Build history of the part. All positions in model axes, mm. Round coordinates to 2 decimals unless told otherwise and drop trailing zeros. Loops run counter-clockwise (first coordinate to the right, second up) from the corner with the lowest first, then second, coordinate; pieces in that order, holes last.
from build123d import *

# Parameters (mm, degrees)
SM_BASE_FLANGE_1_DEPTH      = 1.5
HOLE_WIZARD_M3_1_AT_2_COUNT = 2
HOLE_WIZARD_M3_1_AT_2_PITCH = 60
HOLE_WIZARD_M3_1_AT_3_COUNT = 2
HOLE_WIZARD_M3_1_AT_3_PITCH = 84.852813742
HOLE_WIZARD_M3_1_AT_4_COUNT = 2
HOLE_WIZARD_M3_1_AT_4_PITCH = 60
HOLE_WIZARD_1_D             = 28
HOLE_WIZARD_1_DEPTH         = 100
HOLE_WIZARD_M4_1_D          = 3.3
PATTERN_CIRCULAR_1_COUNT    = 4


# Sheet-metal steps are written as plain solids
with BuildPart() as part:
    # Sketch 1 → 基体-法兰1 (new body)
    with BuildSketch(Plane(origin=(0, 0, 0), x_dir=(0, 0, -1), z_dir=(1, 0, 0))):
        with BuildLine():
            Line((-30, -50), (30, -50))
            ThreePointArc((30, -50), (44.142135624, -44.142135624), (50, -30))
            Line((50, -30), (50, 30))
            ThreePointArc((50, 30), (44.142135624, 44.142135624), (30, 50))
            Line((30, 50), (-30, 50))
            ThreePointArc((-30, 50), (-44.142135624, 44.142135624), (-50, 30))
            Line((-50, 30), (-50, -30))
            ThreePointArc((-50, -30), (-44.142135624, -44.142135624), (-30, -50))
        make_face()
    extrude(amount=-SM_BASE_FLANGE_1_DEPTH)

    # 草图4 → M3 六角凹锥坑头螺钉的锥形沉头孔1 (revolve, cut)
    with BuildSketch(Plane(origin=(-1.5, 30, -30), x_dir=(0, 0, 1), z_dir=(0, 1, 0))):
        Polygon((0, 0), (0, 1.5), (1.7, 1.5), (1.7, 1.77), (3.47, 0), align=None)
    hole_wizard_m3_1 = revolve(axis=Axis((-7.85, 30, -30), (1, 0, 0)), mode=Mode.SUBTRACT)

    # M3 六角凹锥坑头螺钉的锥形沉头孔1 at 2: M3 六角凹锥坑头螺钉的锥形沉头孔1 ×2
    with Locations(*[(0, 0, i * HOLE_WIZARD_M3_1_AT_2_PITCH) for i in range(1, HOLE_WIZARD_M3_1_AT_2_COUNT)]):
        add(hole_wizard_m3_1, mode=Mode.SUBTRACT)

    # M3 六角凹锥坑头螺钉的锥形沉头孔1 at 3: M3 六角凹锥坑头螺钉的锥形沉头孔1 ×2
    with Locations(*[Vector(0, -0.7071067811865476, 0.7071067811865476) * (i * HOLE_WIZARD_M3_1_AT_3_PITCH) for i in range(1, HOLE_WIZARD_M3_1_AT_3_COUNT)]):
        add(hole_wizard_m3_1, mode=Mode.SUBTRACT)

    # M3 六角凹锥坑头螺钉的锥形沉头孔1 at 4: M3 六角凹锥坑头螺钉的锥形沉头孔1 ×2
    with Locations(*[(0, -i * HOLE_WIZARD_M3_1_AT_4_PITCH, 0) for i in range(1, HOLE_WIZARD_M3_1_AT_4_COUNT)]):
        add(hole_wizard_m3_1, mode=Mode.SUBTRACT)

    # 孔1
    with Locations(Plane.ZY.offset(1.5)):
        with Locations((0, 0)):
            Hole(HOLE_WIZARD_1_D / 2, depth=HOLE_WIZARD_1_DEPTH)

    # M4 螺纹孔1 (through all)
    with Locations(Plane.ZY.offset(1.5)):
        with Locations((0, 27.5)):
            hole_wizard_m4_1 = Hole(HOLE_WIZARD_M4_1_D / 2)

    # 阵列(圆周)1: M4 螺纹孔1 ×4 about axis
    pattern_circular_1_axis = Axis((0, 0, 0), (1, 0, 0))
    for i in range(1, PATTERN_CIRCULAR_1_COUNT):
        add(hole_wizard_m4_1.rotate(pattern_circular_1_axis, i * 360 / PATTERN_CIRCULAR_1_COUNT), mode=Mode.SUBTRACT)


solid = part.part
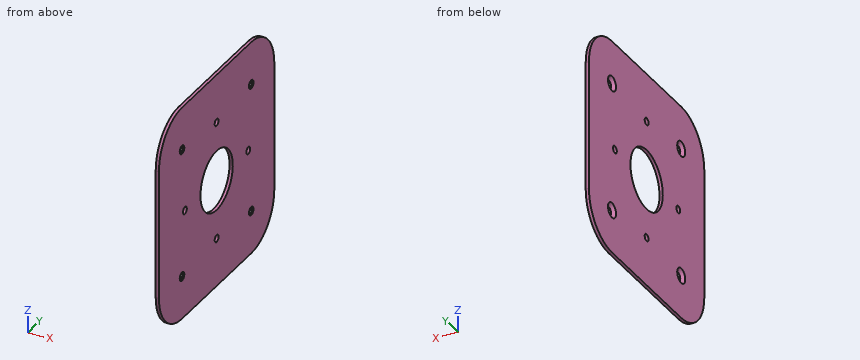
(1) Slice it at A-A on y = 0. List the corners of the cut face in (x, z).
Responses:
outline: (-1.5, -50) - (0, -50) - (0, -29.15) - (-1.5, -29.15) - close; (-1.5, -25.85) - (0, -25.85) - (0, -14) - (-1.5, -14) - close; (-1.5, 14) - (0, 14) - (0, 25.85) - (-1.5, 25.85) - close; (-1.5, 29.15) - (0, 29.15) - (0, 50) - (-1.5, 50) - close
(2) Slice it at C-C on x = -1.25. Count the separate pieces of the cut face and the enclosed holes in it, plus the area to 3 significant figures.
Responses:
separate pieces: 1
enclosed holes: 9
area: 8,880 mm2
(3) Probe line 1 (Y direction, x = -0.5, z = 0); line 2 (Y direction, x = -0.35, z = -27.5); line 3 (Y direction, x = -0.5, z = 1.5). List the from-to ranges inside material, lowest first.
Responses:
line 1: y = -50 to -29.15, -25.85 to -14, 14 to 25.85, 29.15 to 50
line 2: y = -50 to -1.65, 1.65 to 50
line 3: y = -50 to -28.19, -26.81 to -13.92, 13.92 to 26.81, 28.19 to 50
(4) Slice it at D-D on y = -10. List the corners of the cut face in (x, z), plus the area to 3 significant figures.
Responses:
outline: (-1.5, -50) - (0, -50) - (0, -9.8) - (-1.5, -9.8) - close; (-1.5, 9.8) - (0, 9.8) - (0, 50) - (-1.5, 50) - close
area: 121 mm2
